Study the drawing (mm; zero at the part's minimum x, y, z) and answer. Round coordinates to 2 decimals unless told otherwise and drop trailing zeros. Write each loop counter-clockwise with the first axis right and the second up, starting at its lowest first coordinate (ties: lowest second). Pieces come first, ordered by that corner, then holes. Notation, with made-up numbers: M -8,21.5 L 6,21.5 A30 ccw 6,46.5 Z; hole C 25,46.25 d2. An arc over 180 degrees is marked long. Put each result on its own line as item: value. Start each with the question number.
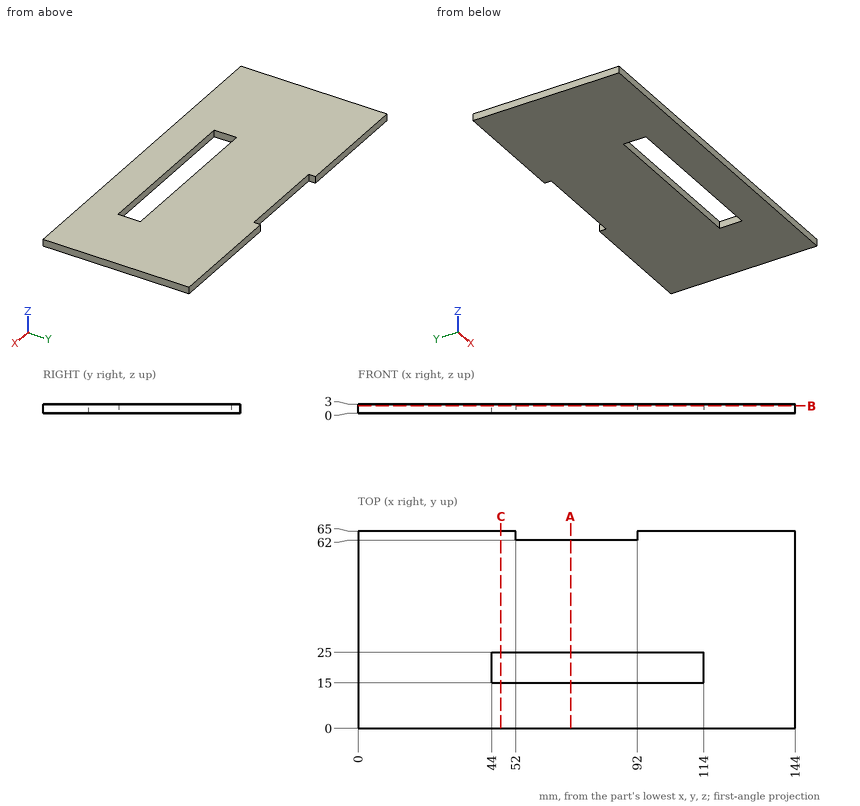
Item 1: Section A-A (x = 70) is taken. Give the vertices of the cut face in (y, z), and give its area (3 significant figures).
Item 2: Section B-B (z = 2.35) is taken. Give the vertices of the cut face in (x, y).
Item 3: Flat-ended cylindrical pins translate along their axes: pin 1 (1.5 mm diameter, centred on x = 90.5, z = 1.5, fed in from +Y); pin 2 (1 mm diameter, centred on y = 10, z = 2.5, fed in from -X). Find the tip coordinate at first contact, or state that the pin passes through.
Item 4: Section C-C (x = 47) is taken. Give the vertices of the cut face in (y, z).
Item 5: Consider line 1 along Y through (x, z) = (45, 0.4); line 2 along Y through (x, z) = (78, 1.75); line 3 along X through (y, z) = (19, 1.3). Determine where each line is inside the solid, lowest interval first. Write a range as [from, to].
Output values:
1. outline: M 0,0 L 15,0 L 15,3 L 0,3 Z; M 25,0 L 62,0 L 62,3 L 25,3 Z
1. area: 156 mm^2
2. outline: M 0,0 L 144,0 L 144,65 L 92,65 L 92,62 L 52,62 L 52,65 L 0,65 Z; hole M 44,15 L 114,15 L 114,25 L 44,25 Z
3. pin 1: stops at y = 62
3. pin 2: stops at x = 0
4. outline: M 0,0 L 15,0 L 15,3 L 0,3 Z; M 25,0 L 65,0 L 65,3 L 25,3 Z
5. line 1: y = [0, 15], [25, 65]
5. line 2: y = [0, 15], [25, 62]
5. line 3: x = [0, 44], [114, 144]
